from build123d import *

# Parameters (mm, degrees)
SKETCH_W        = 118
SKETCH_H        = 52.1
PAD_DEPTH       = 70
SKETCH001_W     = 114
SKETCH001_H     = 50.1
POCKET_DEPTH    = 68
SKETCH002_W     = 50
SKETCH002_H     = 28
POCKET001_DEPTH = 2.001
SKETCH003_R     = 1.5
POCKET002_DEPTH = 2.001
SKETCH004_R     = 3
SKETCH004_R_2   = 1.5
PAD001_DEPTH    = 5
SKETCH005_R     = 2.2
POCKET003_DEPTH = 118.001
POCKET004_DEPTH = 2.001
FILLET_R        = 4
FILLET001_R     = 4


with BuildPart() as part:
    # Sketch → Pad (new body)
    with BuildSketch(Plane.XY):
        Rectangle(SKETCH_W, SKETCH_H)
    extrude(amount=PAD_DEPTH)

    # Sketch001 → Pocket (cut)
    with BuildSketch(Plane.XY.offset(70)):
        with Locations((0, -1)):
            Rectangle(SKETCH001_W, SKETCH001_H)
    extrude(amount=-POCKET_DEPTH, mode=Mode.SUBTRACT)

    # Sketch002 → Pocket001 (cut, through all)
    with BuildSketch(Plane.XY.offset(2)):
        with Locations((-25, -2)):
            Rectangle(SKETCH002_W, SKETCH002_H)
    extrude(amount=-POCKET001_DEPTH, mode=Mode.SUBTRACT)

    # Sketch003 → Pocket002 (cut, through all)
    with BuildSketch(Plane.XY.offset(2)):
        with Locations((-26, 17.7)):
            Circle(SKETCH003_R)
        with Locations((-26, -21.7)):
            Circle(SKETCH003_R)
    extrude(amount=-POCKET002_DEPTH, mode=Mode.SUBTRACT)

    # Sketch004 → Pad001 (new body)
    with BuildSketch(Plane.XY.offset(2)):
        with Locations((-26, 17.7)):
            Circle(SKETCH004_R)
        with Locations((-26, 17.7)):
            Circle(SKETCH004_R_2, mode=Mode.SUBTRACT)
        with Locations((-26, -21.7)):
            Circle(SKETCH004_R)
        with Locations((-26, -21.7)):
            Circle(SKETCH004_R_2, mode=Mode.SUBTRACT)
    extrude(amount=PAD001_DEPTH)

    # Sketch005 → Pocket003 (cut, through all)
    with BuildSketch(Plane(origin=(-59, 0, 0), x_dir=(0, -1, 0), z_dir=(-1, 0, 0))):
        with Locations((-10.85, 65)):
            Circle(SKETCH005_R)
        with Locations((14.15, 65)):
            Circle(SKETCH005_R)
    extrude(amount=-POCKET003_DEPTH, mode=Mode.SUBTRACT)

    # Sketch006 → Pocket004 (cut, through all)
    with BuildSketch(Plane.XY.offset(2)):
        with BuildLine():
            Line((35, -16.05), (35, -26.05))
            Line((35, -26.05), (25, -26.05))
            Line((25, -26.05), (25, -16.05))
            ThreePointArc((35, -16.05), (30, -11.049989), (25, -16.05))
        make_face()
    extrude(amount=-POCKET004_DEPTH, mode=Mode.SUBTRACT)

    # Fillet
    fillet_edges = [part.edges().sort_by_distance(p)[0] for p in [
        (0, 24.05, 2),
        (-57, -1, 2),
        (57, -1, 2),
    ]]
    fillet(fillet_edges, radius=FILLET_R)

    # Fillet001
    fillet001_edges = [part.edges().sort_by_distance(p)[0] for p in [
        (-59, 0, 0),
        (0, 26.05, 0),
        (59, 0, 0),
    ]]
    fillet(fillet001_edges, radius=FILLET001_R)


solid = part.part
Check sheet for the modelled part. Datum: model origin and axes. Units: mm. A direction names the side the tool comes from. Round coordinates to 2 decimals unless told otherwise and drop trailing zeros. Order: outer loops, then holes, each group sorted by start corner. A loop starts at its lowest first (then second) coordinate and runs counter-clockwise, first axis right, second up. Notation, with made-up numbers: M 52,-26 L 76,-26 A20 ccw 76,13 Z; hole C 81,50.5 d4. An arc over 180 degrees is marked long. One line per item, written item: value. Start each with the question number.
1. Release check for a two-part mould opening along X. For faces 1 (the flat face through (59, 0, 37)), 2 (the cylindrical face through (-58.01, 12.47, 66.49)), 3 (the cylindrical face through (-57.797, 0.365, 1.141)), 4 (the flat face through (-25, 16, 7)) record: released by +X, released by -X, zero draft, split by the parting line, or undercut.
2. Section check A-A on z = 65. Enter the section's corners in (x, y), and give its area (3 significant figures).
3. Section check D-D on z = 56.5. Enter the section's corners in (x, y).
4. Section check B-B on y = 6.5. Enter the section's corners in (x, z).
5. Section check C-C on x = -38.5. Enter the section's corners in (y, z), and give its area (3 significant figures).
6. Gauge pin test, flat ends, axial feed: P1, Ø1, axis at x = -36, z = 1, coming from the +Y side; P2, Ø6, axis at x = 2.5, z = 21.5, coming from the -Y side; P3, Ø2.5, axis at x = -26, y = 17.7, coming from the -Z side; P4, Ø5, axis at x = -43, y = 15.5, coming from the +Z side. Record the tip position at first contact, or that the pin passes through.
7. Access from +Z, -Z, +X, -X, +Y, -Y to the whole of each face (thin tool, end or side, straight path). Record for faces 5 (the cylindrical face through (-28.21, -19.67, 4.46)), 6 (the flat face through (57, -1, 38)), 7 (the cylindrical face through (57.99, 12.47, 66.49)).
8. Scan lines: line 1 along X through (y, z) = (1.5, 57); line 2 along Y through (x, z) = (30, 55); line 3 along Z through (x, y) = (17, -21). Record each from-to range of solid material in increasing order.
Results found:
1. face 1: released by +X
1. face 2: zero draft
1. face 3: released by -X
1. face 4: undercut
2. outline: M -59,-26.05 L -57,-26.05 L -57,-16.35 L -59,-16.35 Z; M -59,-11.95 L -57,-11.95 L -57,8.65 L -59,8.65 Z; M -59,13.05 L -57,13.05 L -57,24.05 L 57,24.05 L 57,13.05 L 59,13.05 L 59,26.05 L -59,26.05 Z; M 57,-26.05 L 59,-26.05 L 59,-16.35 L 57,-16.35 Z; M 57,-11.95 L 59,-11.95 L 59,8.65 L 57,8.65 Z
2. area: 401 mm^2
3. outline: M -59,-26.05 L -57,-26.05 L -57,24.05 L 57,24.05 L 57,-26.05 L 59,-26.05 L 59,26.05 L -59,26.05 Z
4. outline: M -59,4 A4 ccw -55,0 L -50,0 L -50,2 L -53,2 A4 cw -57,6 L -57,70 L -59,70 Z; M 0,0 L 55,0 A4 ccw 59,4 L 59,70 L 57,70 L 57,6 A4 cw 53,2 L 0,2 Z
5. outline: M -26.05,0 L -16,0 L -16,2 L -26.05,2 Z; M 12,0 L 22.05,0 A4 ccw 26.05,4 L 26.05,70 L 24.05,70 L 24.05,6 A4 cw 20.05,2 L 12,2 Z
5. area: 184 mm^2
6. P1: y = 25.17
6. P2: y = 24.05
6. P3: through
6. P4: z = 2
7. face 5: +Z
7. face 6: +Z, -Y
7. face 7: +X, -X
8. line 1: -59 to -57, 57 to 59
8. line 2: 24.05 to 26.05
8. line 3: 0 to 2
